```python
from build123d import *

# Parameters (mm, degrees)
F0_R     = 50.8
F1_DEPTH = 25.4
F3_D     = 10.71626
F3_DEPTH = 22.225
F3_TIP   = 3.2194893086


with BuildPart() as f1:
    # F0 (on Front) → F1 (new body)
    with BuildSketch(Plane.XZ):
        Circle(F0_R)
    extrude(amount=F1_DEPTH)

    # F3
    with Locations(Plane.XZ.offset(25.4)):
        with Locations((-38.0981450941, 0.3759526402), (-18.7234880101, 33.1819378087), (19.3746570841, 32.8059851685), (38.0981450941, -0.3759526402), (18.7234880101, -33.1819378087), (-19.3746570841, -32.8059851685)):
            Hole(F3_D / 2, depth=F3_DEPTH)
            with Locations((0, 0, -(F3_DEPTH + F3_TIP / 2))):  # 118° drill point
                Cone(0, F3_D / 2, F3_TIP, mode=Mode.SUBTRACT)


solid = f1.part
```
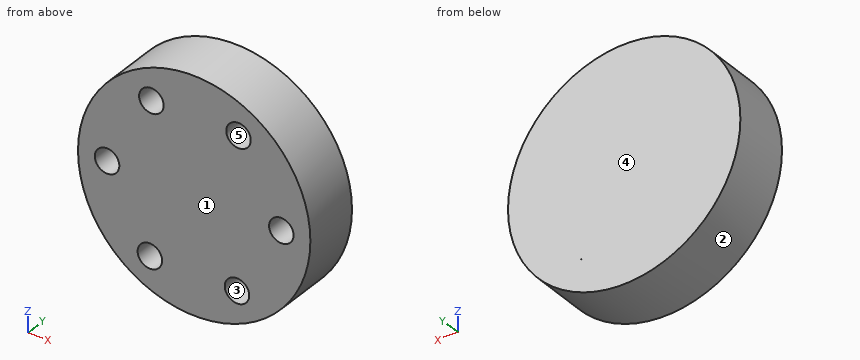
Design review of the part built by this model. Coordinates are the model's own, in mm. Face numbers are marked on the shaded views. A direction names the side the tool comes from. Round coordinates to 2 decimals unless told otherwise and drop trailing zeros. Write each loop counter-clockwise with the first axis right and the second up, starting at its lowest first coordinate (ties: lowest second). Pieces come first, ordered by that corner, then holes.
Item 1: For the marked faces 4 and 5, list the 3-axis set-ups (+Z, -Z, +X, -X, +Y, -Y) from which the entire face can be reached by the end or side of a thin tool; tool diameter is ignored.
Item 2: The part is to be moulded in two halves that separate along X. For the marked faces 1, 2 and 3, say which applies: +X half, -X half, draft (parallel to the pull), parting line (faces both ways), or undercut.
Item 3: We need section C-C on z = 21. Write out the cut boundary in (x, y).
Item 4: We need section B-B on x = -11. Write out the cut boundary in (y, z), and give its area (3 significant figures).
Item 5: For probe 1 along X at (y, z) = (-22.75, -37); probe 2 along X at (y, z) = (-15.25, 31); probe 3 along Z at (x, y) = (19, -23.5), list the stretches that pass through material, from the lowest coordinate up.
Item 6: We need section A-A on y = -22. Write out the cut boundary in (x, z).
Item 7: Clearance check with flat-ended pins moving along their axes: pin 1 Ø1.5 at (x, y) = (6, -14.5) entering from -Z; pin 2 Ø4 at (y, z) = (-20.5, -32.5) entering from +X (3 decimals); pin 3 Ø2 at (x, y) = (-20.5, -3.5) entering from +Z. State where each tip first meets the part, or that it passes through.
Returned:
1. face 4: +Z, -Z, +X, -X, +Y
1. face 5: -Y
2. face 1: draft
2. face 2: parting line
2. face 3: undercut
3. outline: (-46.26, -25.4) - (46.26, -25.4) - (46.26, 0) - (-46.26, 0) - close
4. outline: (-25.4, -49.59) - (0, -49.59) - (0, 49.59) - (-25.4, 49.59) - close
4. area: 2,520 mm2
5. probe 1: x = -34.81 to -22.71, -16.04 to 14.96, 22.48 to 34.81
5. probe 2: x = -40.24 to -23.62, -13.83 to 14.33, 24.42 to 40.24
5. probe 3: z = -47.11 to -38.53, -27.83 to 27.46, 38.15 to 47.11
6. outline: circle Ø101.6 at (0, 0); hole circle Ø10.72 at (-38.1, 0.38); hole circle Ø10.72 at (-19.37, -32.81); hole circle Ø10.72 at (-18.72, 33.18); hole circle Ø10.72 at (18.72, -33.18); hole circle Ø10.72 at (19.37, 32.81); hole circle Ø10.72 at (38.1, -0.38)
7. pin 1: stops at z = -50.53
7. pin 2: stops at x = 40.625
7. pin 3: stops at z = 46.91
